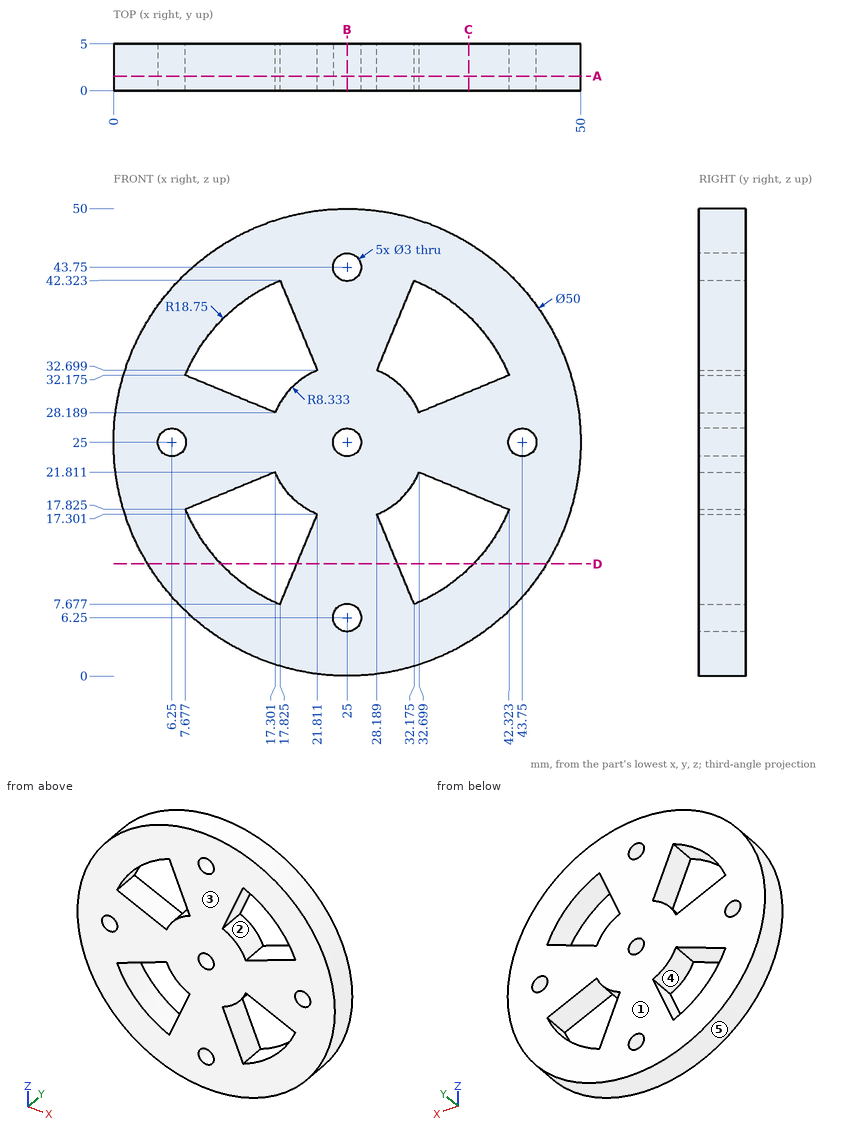
For this review, use the dimensioned drawing (mm, ordinates from the lowest corner) and the shaded views. A direction names the side the tool comes from. Coordinates: 2 decimals unless noted, no trailing zeros. Order: outer loops, then holes, each group sorted by start corner. A loop starts at its lowest first (then second) coordinate and runs counter-clockwise, first axis right, second up. Notation, with made-up numbers: (44, -11.5) - (55, -11.5) arc R23 cw to (55, 24.5) - close; hole circle Ø6 at (44.25, 71). An arc over 180 degrees is marked (long way). Answer as a JSON object with one key per item and string values. Group by question number.
1. We need section C-C on x = 38. State the section outline as (y, z) points (1 decimal), then the cut area to 3 significant figures.
2. Clearance check with flat-ended pins moving along their axes: P1, Ø8, axis at x = 28, z = 41, coming from the -Y side; P2, Ø3, axis at y = 2.5, z = 42.5, coming from the -X side; P3, Ø2, axis at y = 1, z = 8, coming from the +X side; P4, Ø3, axis at x = 22.5, y = 2.5, coming from the +Z side. State where each tip first meets the part, or that it passes through.
3. For probe 1 along Z at (x, y) = (25, 2.7); probe 2 along X at (y, z) = (0.5, 25.5) (1 decimal), list the stretches that pass through material, from the lowest coordinate up.
4. We need section D-D on z = 12. State the section outline as (x, y) points (1 decimal).
5. We need section B-B on x = 25. State the section outline as (y, z) points.
6. We need section A-A on y = 1.55. Give the number of separate pieces and of enclosed holes in the cut face, then the cut area to 4 significant figures.
7. For the marked faces 1 and 2, list the 3-axis set-ups (+Z, -Z, +X, -X, +Y, -Y) from which the entire face can be reached by the end or side of a thin tool; tool diameter is ignored.
8. The part is to be moulded in two halves that separate along X. For the marked faces 3, 4 and 5, say which applies: pulls with the +X half, pulls with the -X half, needs draft (parallel to the pull), parting line crosses it, or undercut.
Final values:
{
 "1": {"outline": "(0, 3.6) - (5, 3.6) - (5, 11.5) - (0, 11.5) - close; (0, 19.6) - (5, 19.6) - (5, 30.4) - (0, 30.4) - close; (0, 38.5) - (5, 38.5) - (5, 46.4) - (0, 46.4) - close", "area": "132 mm²"},
 "2": {"P1": "y = 0", "P2": "x = 5.79", "P3": "x = 44.21", "P4": "z = 49.98"},
 "3": {"probe 1": "0 to 4.75, 7.75 to 23.5, 26.5 to 42.25, 45.25 to 50", "probe 2": "0 to 4.8, 7.7 to 23.6, 26.4 to 42.3, 45.2 to 50"},
 "4": {"outline": "(3.6, 0) - (11.5, 0) - (11.5, 5) - (3.6, 5) - close; (19.6, 0) - (30.4, 0) - (30.4, 5) - (19.6, 5) - close; (38.5, 0) - (46.4, 0) - (46.4, 5) - (38.5, 5) - close"},
 "5": {"outline": "(0, 0) - (5, 0) - (5, 4.75) - (0, 4.75) - close; (0, 7.75) - (5, 7.75) - (5, 23.5) - (0, 23.5) - close; (0, 26.5) - (5, 26.5) - (5, 42.25) - (0, 42.25) - close; (0, 45.25) - (5, 45.25) - (5, 50) - (0, 50) - close"},
 "6": {"separate pieces": "1", "enclosed holes": "9", "area": "1,485 mm²"},
 "7": {"face 1": "+Z, -Z, +X, -X, +Y", "face 2": "+Y, -Y"},
 "8": {"face 3": "needs draft", "face 4": "undercut", "face 5": "parting line crosses it"}
}
